For this review, take the finished solid that the model builds, in its own axes (mm). A direction names the side the tool comes from. Give positions to 0.01 mm unless a question says otherwise; leave off trailing zeros. Order: outer loops, then holes, each group sorted by start corner. A loop starts at its lowest first (then second) coordinate and runs counter-clockwise, first axis right, second up.
Item 1: Consider section A-A (y = 0). Give the boundary of the cut face in (x, z), plus the area to 3 significant figures.
Item 2: Consider section D-D (x = -3.5). Give the number of separate pieces and of enclosed holes in the cut face, plus the area to 3 significant figures.
Item 3: The part is to be moulded in two halves that separate along Z. For faces 5 (the flat face through (-0.06, -5.41, 6.87)), 6 (the flat face through (-0.06, 6.87, -5.41)), 7 (the flat face through (-0.06, 5.41, -6.87)), 8 (the flat face through (4, 0, 9)), say which applies: released by +Z, released by -Z, zero draft, split by the parting line, or undercut.
Item 4: Machinability: for faces 1 (the flat face through (4, 8, -4)), 2 (the flat face through (0, 1.25, -9)), 3 (the flat face through (0, 9, 1.25)), 4 (the flat face through (-0.06, -6.87, -5.41)), which of the approach directions +Z, -Z, +X, -X, +Y, -Y give a long, thin tool a straight path to every point of the face, cutting with its end or side? Answer none if there is none.
Item 5: Consider section C-C (y = 2). Give the boundary of the cut face in (x, z), plus the area to 3 significant figures.
Item 6: For P1, Ø1.7, axis at x = 1, y = 8.5, coming from the -Z side; P2, Ø0.8, axis at x = 0.5, z = -8.5, coming from the -Y side; P3, Ø5, axis at y = -3, z = 1.5, coming from the -X side; P4, Ø3, axis at x = -2, z = 7, coming from the -Y side, all flat-tipped, find the tip position at first contact; note any pin that passes through.
Item 7: For probe 1 along X at (y, z) = (5, -7); probe 2 along Z at (x, y) = (-2.5, -6.5); probe 3 along Y at (x, z) = (-1, 8.25), list the stretches that pass through material, from the lowest coordinate up.
```python
from build123d import *

# Parameters (mm, degrees)
ESQUISSE1_W                  = 10
ESQUISSE1_H                  = 1.5
ESQUISSE2_W                  = 8
ESQUISSE2_H                  = 2.5
ENL_V_MAT_EXTRU_1_DEPTH      = 10.5
R_P_TITION_CIRCULAIRE1_COUNT = 12


with BuildPart() as part:
    # Esquisse1 → Base-Révolution (revolve)
    with BuildSketch(Plane.XY):
        with Locations((0, 8.75)):
            Rectangle(ESQUISSE1_W, ESQUISSE1_H)
    revolve(axis=Axis((11.7, 0, 0), (-1, 0, 0)))

    # Esquisse2 → Enlèv. mat.-Extru.1 (cut, through all)
    with BuildSketch(Plane.XY):
        Rectangle(ESQUISSE2_W, ESQUISSE2_H)
    enl_v_mat_extru_1 = extrude(amount=-ENL_V_MAT_EXTRU_1_DEPTH, mode=Mode.SUBTRACT)

    # Répétition circulaire1: Enlèv. mat.-Extru.1 ×12 about axis
    r_p_tition_circulaire1_axis = Axis((-50, 0, 0), (1, 0, 0))
    for i in range(1, R_P_TITION_CIRCULAIRE1_COUNT):
        add(enl_v_mat_extru_1.rotate(r_p_tition_circulaire1_axis, i * 360 / R_P_TITION_CIRCULAIRE1_COUNT), mode=Mode.SUBTRACT)


solid = part.part
```
Resolved:
1. outline: (-5, -9.5) - (-4, -9.5) - (-4, -8) - (-5, -8) - close; (-5, 8) - (-4, 8) - (-4, 9.5) - (-5, 9.5) - close; (4, -9.5) - (5, -9.5) - (5, -8) - (4, -8) - close; (4, 8) - (5, 8) - (5, 9.5) - (4, 9.5) - close
1. area: 6.00 mm2
2. separate pieces: 12
2. enclosed holes: 0
2. area: 37.3 mm2
3. face 5: released by +Z
3. face 6: undercut
3. face 7: released by -Z
3. face 8: zero draft
4. face 1: none
4. face 2: +Z, -Z
4. face 3: +Y, -Y
4. face 4: -Y
5. outline: (-5, -9.29) - (5, -9.29) - (5, -7.75) - (-5, -7.75) - close; (-5, 7.75) - (5, 7.75) - (5, 9.29) - (-5, 9.29) - close
5. area: 30.8 mm2
6. P1: stops at z = -3.63
6. P2: stops at y = -3.63
6. P3: passes through
6. P4: stops at y = -7.53
7. probe 1: x = -5 to -4, 4 to 5
7. probe 2: z = -6.93 to -5.2, 5.2 to 6.93
7. probe 3: y = -3.32 to -1.25, 1.25 to 3.32
